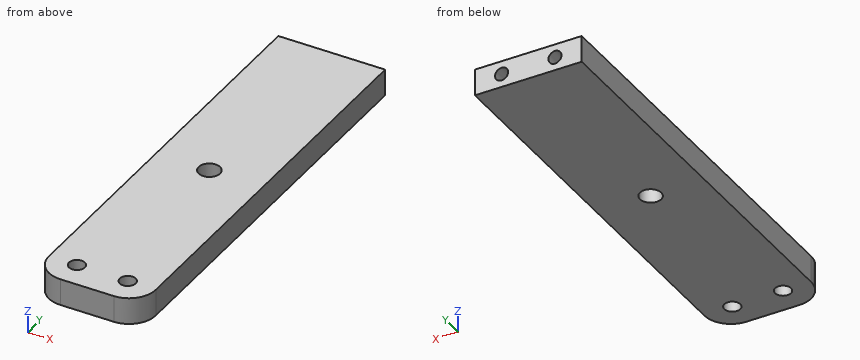
Autodesk Inventor part; units mm, degrees
ref_plane "YZ Plane" through (0, 0, 0) normal (1, 0, 0) x (0, 1, 0)
ref_plane "XZ Plane" through (0, 0, 0) normal (0, 1, 0) x (-1, 0, 0)
ref_plane "XY Plane" through (0, 0, 0) normal (0, 0, 1) x (1, 0, 0)
sketch "Sketch1" plane through (0, 0, 0) normal (0, 0, 1) x (1, 0, 0)
  line L0 (40, 0) -> (60, 0)
  line L1 (60, 0) -> (60, -80)
  line L2 (60, -80) -> (40, -80)
  line L3 (40, -80) -> (40, 0)
  point P0 (0, 0)
  dimension "d0" = 40
  dimension "d1" = 20
  dimension "d2" = 80
extrude "Extrusion1" add sketch "Sketch1" along normal blind 5
sketch "Sketch2" plane through (0, 0, 5) normal (0, 0, 1) x (1, 0, 0)
  circle A0 centre (45.25, -75) radius 1.5
  circle A1 centre (54.75, -75) radius 1.5
  line L0 (40, -80) -> (60, -80)
  line L1 (60, -80) -> (60, 0)
  point P0 (0, 0)
  dimension "d5" = 9.5
  dimension "d6" = 5
  dimension "d7" = 5
  dimension "d8" = 5.25
  dimension "d9" = 3
  dimension "d10" = 3
hole "Hole1" at (45.25, -75, 5) at (54.75, -75, 5) direction (0, 0, -1) diameter 3 depth 20 tip angle 118
fillet "Fillet1" radius 5 2 edges at (40, -80, 2.5) (60, -80, 2.5)
sketch "Sketch4" plane through (0, 0, 5) normal (0, 0, 1) x (1, 0, 0)
  circle A0 centre (50, -40) radius 2
  line L0 (40, 0) -> (40, -75)
  line L1 (60, 0) -> (40, 0)
  line L2 (45, -80) -> (55, -80)
  point P0 (0, 0)
  point P1 (40, -73.521)
  dimension "d32" = 4
  dimension "d33" = 10
  dimension "d34" = 40
  dimension "d42" = 80
hole "Hole3" at (50, -40, 5) direction (0, 0, -1) diameter 4 depth 20 tip angle 118
sketch "Sketch6" plane through (40, 0, 0) normal (0, 1, 0) x (1, 0, 0)
  line L0 (5, 0) -> (5, -5)
  circle A0 centre (5, -2.5) radius 1.5
  line L1 (15, -5) -> (15, 0)
  circle A1 centre (15, -2.5) radius 1.5513
  point P0 (-40, 0)
  dimension "d50" = 3.1027
  dimension "d51" = 3
hole "Hole5" at (45, 0, 2.5) at (55, 0, 2.5) direction (0, -1, 0) diameter 2.459 depth 30 tip angle 118
equation "\"d11\" = d9"
equation "\"d34\" = 0.5 * d42"
equation "\"d35\" = d32"
properties part number "Z-Endstophalter2"
The model under review builds one solid part; all positions refer to its coordinate system, in mm. Round coordinates to 2 decimals unless told otherwise and drop trailing zeros. Write each loop counter-clockwise with the first axis right and the second up, starting at its lowest first coordinate (ties: lowest second). Pieces come first, ordered by that corner, then holes. Notation, with made-up numbers: (74.25, 5.5) - (102.25, 5.5) arc R23 cw to (102.25, 15.5) - close; hole circle Ø9 at (36, -35). An arc over 180 degrees is marked (long way). Answer as CSV lines item,"result". Start each with the question number.
(1) We need section D-D on x = 59. State the section outline as (y, z) points.
(2) We need section C-C on y = -7.5. State the section outline as (x, z) points, plus the area to 3 significant figures.
(3) We need section A-A on x = 50. State the section outline as (y, z) points.
(4) To check wall thickness, follow line 1 (X direction, y = -16.5, z = 2.5); line 2 (X direction, y = -75, z = 2.15); line 3 (Z direction, x = 45, y = -7.75). State the ranges of each line that lie inside material, in increasing order.
(5) For pin 1 Ø1 at (x, z) = (57.5, 3) entering from -Y; pin 2 Ø2 at (x, z) = (45, 2.5) entering from +Y, all flat-tipped, find the tip position at first contact; note any pin that passes through.
(6) We need section B-B on y = -40. State the section outline as (x, z) points.
Worked answers:
1,outline,"(-78, 0) - (0, 0) - (0, 5) - (-78, 5) - close"
2,outline,"(40, 0) - (60, 0) - (60, 5) - (40, 5) - close; hole circle Ø2.46 at (45, 2.5); hole circle Ø2.46 at (55, 2.5)"
2,area,"90.5 mm²"
3,outline,"(-80, 0) - (-42, 0) - (-42, 5) - (-80, 5) - close; (-38, 0) - (0, 0) - (0, 5) - (-38, 5) - close"
4,line 1,"40 to 43.77, 46.23 to 53.77, 56.23 to 60"
4,line 2,"40 to 43.75, 46.75 to 53.25, 56.25 to 60"
4,line 3,"0 to 1.27, 3.73 to 5"
5,pin 1,"y = -79.58"
5,pin 2,"y = -30.14"
6,outline,"(40, 0) - (48, 0) - (48, 5) - (40, 5) - close; (52, 0) - (60, 0) - (60, 5) - (52, 5) - close"
